Design review of the part shown in the three views and the two pictorial views. Dimensions are in mm from the part's minimum x, y and z. Round coordinates to 2 decimals unless told otherwise and drop trailing zeros. Loops run counter-clockwise (first coordinate to the right, second up) from the corner with the lowest first, then second, coordinate; pieces in that order, holes last. Notation, with made-up numbers: (81, 46) -> (89, 46) arc R13 ccw to (89, 71) -> close; hole circle Ø9 at (60, -4). An arc over 180 degrees is marked (long way). Use a Markdown table: item, result. Add a question column.
1) Consider section B-B on x = 3.25. Give the boundary of the cut face in (y, z), plus the area to 3 significant figures.
2) Consider section D-D on y = 7.75. Give the boundary of the cut face in (x, z).
3) Mouldability with a two-part tool opening along Z and no side actions: class the marked faces 1, 2 and 3 as released by +Z, released by -Z, zero draft, split by the parting line, or undercut.
4) Consider section A-A on z = 3.25. Give the boundary of the cut face in (x, y), plus the area to 3 significant figures.
5) Wall thickness on probe 1 along Y at (x, z) = (3, 3.25); probe 2 along Z at (x, y) = (3.25, 26); probe 3 along Z at (x, y) = (2, 26): over which ranges is each line inside the solid? List them lowest first.
6) Consider section C-C on y = 26. Give the boundary of the cut face in (x, z).
7) Insertion check: pin 1 (2 mm diameter, centred on y = 9, z = 4.5, fed in from +X); pin 2 (2 mm diameter, centred on x = 1.5, y = 7.5, fed in from +Z). Each pin has a flat end and moves straight along its axis. Give the tip position at first contact, or say it passes through.
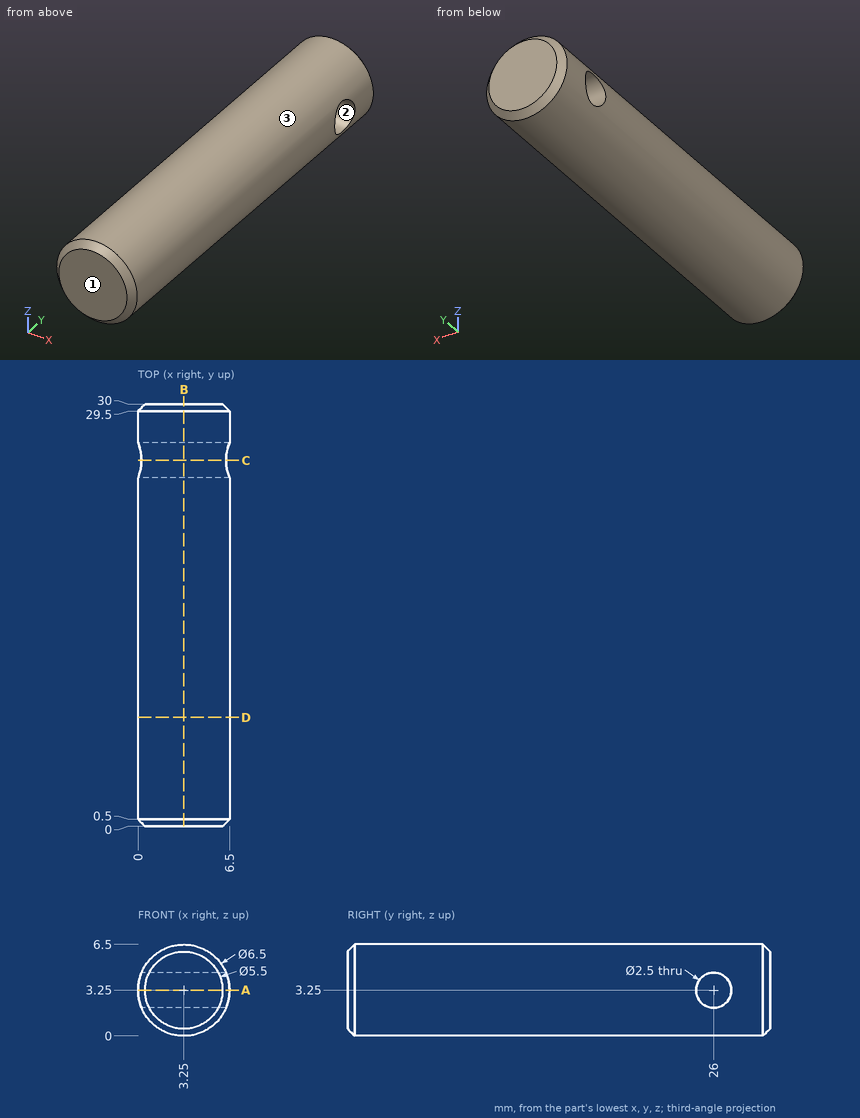
Result set:
| question | item | result |
|---|---|---|
| 1 | outline | (0, 0.5) -> (0.5, 0) -> (29.5, 0) -> (30, 0.5) -> (30, 6) -> (29.5, 6.5) -> (0.5, 6.5) -> (0, 6) -> close; hole circle Ø2.5 at (26, 3.25) |
| 1 | area | 190 mm2 |
| 2 | outline | circle Ø6.5 at (3.25, 3.25) |
| 3 | face 1 | zero draft |
| 3 | face 2 | undercut |
| 3 | face 3 | split by the parting line |
| 4 | outline | (0, 0.5) -> (0.5, 0) -> (6, 0) -> (6.5, 0.5) -> (6.5, 24.75) -> (0, 24.75) -> close; (0, 27.25) -> (6.5, 27.25) -> (6.5, 29.5) -> (6, 30) -> (0.5, 30) -> (0, 29.5) -> close |
| 4 | area | 178 mm2 |
| 5 | probe 1 | 0 to 24.75, 27.25 to 30 |
| 5 | probe 2 | 0 to 2, 4.5 to 6.5 |
| 5 | probe 3 | 0.25 to 2, 4.5 to 6.25 |
| 6 | outline | (0.25, 2) arc R3.25 ccw to (6.25, 2) -> close; (0.25, 4.5) -> (6.25, 4.5) arc R3.25 ccw to start |
| 7 | pin 1 | x = 6.49 |
| 7 | pin 2 | z = 6.41 |
